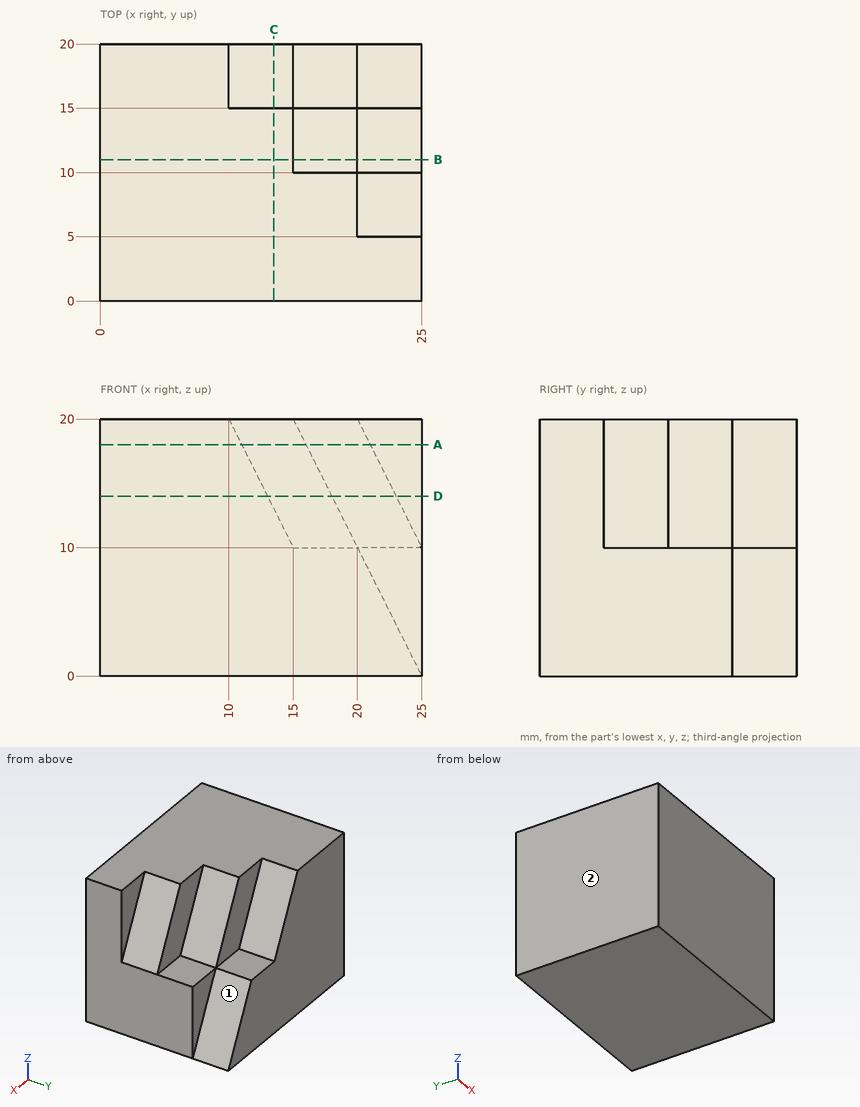
Study the drawing (mm; zero at the part's minimum x, y, z) and answer. A direction names the side the tool comes from. Coordinates: 2 decimals unless noted, no trailing zeros. Write each loop counter-clockwise with the first axis right and the second up, starting at its lowest first coordinate (ties: lowest second). Pieces come first, ordered by that corner, then holes. Notation, with made-up numbers: (41, -30.75) - (66, -30.75) arc R33 cw to (66, 7.25) - close; hole circle Ø8 at (-5, -19). An arc over 180 degrees is marked (long way). Answer as a JSON object with one key per item and string values. Group by question number.
1. Which of the six approach directions +Z, -Z, +X, -X, +Y, -Y give full straight-line access (tool end or side, diameter ignored) to the marked faces 1 and 2?
2. A cutting plane is placed at A-A (z = 18). Determine the outline of the cut face in (x, y).
3. Each of these flat-tipped pins is pushed along its axis until it touches: P1, Ø5, axis at x = 14, z = 14.5, coming from the +Y side; P2, Ø5.5, axis at x = 23.5, z = 17.5, coming from the +Y side; P3, Ø4, axis at x = 23.5, y = 12.5, coming from the +Z side; P4, Ø1, axis at y = 16, z = 7, coming from the +X side. Where does it stop, or does it pass through?
4. A cutting plane is placed at C-C (x = 13.5). Determine the outline of the cut face in (y, z), plus the area to 3 significant figures.
5. A cutting plane is placed at B-B (y = 11). Determine the outline of the cut face in (x, z).
6. A cutting plane is placed at D-D (z = 14). Determine the outline of the cut face in (x, y), plus the area to 3 significant figures.
7. Consider L1, parallel to Z at x = 16, y = 19.25; L2, parallel to Y at x = 16.75, z = 14; L3, parallel to Z at x = 22.5, y = 17. Determine where each line is inside the solid, lowest interval first. Write a range as [from, to].
Worked out:
{
 "1": {"face 1": "+Z, +X, +Y", "face 2": "+Z, -Z, -X, +Y, -Y"},
 "2": {"outline": "(0, 0) - (25, 0) - (25, 5) - (21, 5) - (21, 10) - (16, 10) - (16, 15) - (11, 15) - (11, 20) - (0, 20) - close"},
 "3": {"P1": "stops at y = 20", "P2": "stops at y = 10", "P3": "stops at z = 10", "P4": "stops at x = 21.75"},
 "4": {"outline": "(0, 0) - (20, 0) - (20, 13) - (15, 13) - (15, 20) - (0, 20) - close", "area": "365 mm²"},
 "5": {"outline": "(0, 0) - (25, 0) - (25, 10) - (20, 10) - (15, 20) - (0, 20) - close"},
 "6": {"outline": "(0, 0) - (25, 0) - (25, 5) - (23, 5) - (23, 10) - (18, 10) - (18, 15) - (13, 15) - (13, 20) - (0, 20) - close", "area": "395 mm²"},
 "7": {"L1": "z = [0, 10]", "L2": "y = [0, 15]", "L3": "z = [0, 5]"}
}
